from build123d import *

# Parameters (mm, degrees)
BOSS_EXTRUDE1_DEPTH     = 40
CUT_EXTRUDE1_DEPTH      = 40
SKETCH3_W               = 4.376715803
SKETCH3_H               = 7.921330006
BOSS_EXTRUDE2_DEPTH     = 40
CUT_EXTRUDE2_DEPTH      = 78.145313728
CUT_EXTRUDE2_DEPTH_BACK = 78.145313728
CUT_EXTRUDE3_DEPTH      = 40
CUT_EXTRUDE4_DEPTH      = 43.935998882
CUT_EXTRUDE4_DEPTH_BACK = 43.935998882
SKETCH6_R               = 2
CUT_EXTRUDE5_DEPTH      = 5
SKETCH8_R               = 5
CUT_EXTRUDE6_DEPTH      = 5
CUT_EXTRUDE7_START      = -2
SKETCH9_W               = 6.222682415
SKETCH9_H               = 53.403341902
CUT_EXTRUDE7_DEPTH      = 16


with BuildPart() as part:
    # Sketch1 → Boss-Extrude1 (new body)
    with BuildSketch(Plane(origin=(0, 0, 0), x_dir=(1, 0, 0), z_dir=(0, 1, 0))):
        Polygon((-35, 12.5), (-20.56624327, -12.5), (35, -12.5), (35, 12.5), align=None)
    extrude(amount=BOSS_EXTRUDE1_DEPTH)

    # Sketch2 → Cut-Extrude1 (cut)
    with BuildSketch(Plane.XY.offset(12.5)):
        Polygon((-20.56624327, 40), (35, 32.5), (35, 40), align=None)
        Polygon((35, 7.5), (-20.56624327, 0), (35, 0), align=None)
    extrude(amount=-CUT_EXTRUDE1_DEPTH, mode=Mode.SUBTRACT)

    # Sketch3 → Boss-Extrude2 (add)
    with BuildSketch(Plane(origin=(-20.837341226, 0, 12.030444566), x_dir=(0.4999999999999981, 0, 0.8660254037844397), z_dir=(-0.8660254037844398, 0, 0.4999999999999982))):
        with Locations((-10.675795445, 21.421253709)):
            Rectangle(SKETCH3_W, SKETCH3_H)
    extrude(amount=BOSS_EXTRUDE2_DEPTH)

    # Sketch4 → Cut-Extrude2 (cut, two sides: drawn at the far end of the back side and taken through both)
    with BuildSketch(Plane(origin=(-4.243718771, 0, -7.350336525), x_dir=(0.8660254037844397, 0, -0.4999999999999983), z_dir=(0.4999999999999982, 0, 0.8660254037844396)).offset(-CUT_EXTRUDE2_DEPTH_BACK)):
        with BuildLine():
            Line((-25.260889132, 35.934120187), (-19.597573928, 35.934120187))
            ThreePointArc((-19.597573928, 35.934120187), (-17.574079433, 36.729704946), (-16.260889132, 34.996783621))
            Line((-16.260889132, 34.996783621), (-16.260889132, 27.623217913))
            ThreePointArc((-16.260889132, 27.623217913), (-14.610889132, 19.996783621), (-16.260889132, 12.37034933))
            Line((-16.260889132, 12.37034933), (-16.260889132, 4.996783621))
            ThreePointArc((-16.260889132, 4.996783621), (-17.574079433, 3.263862297), (-19.597573928, 4.059447055))
            Line((-19.597573928, 4.059447055), (-25.260889132, 4.059447055))
            Line((-25.260889132, 4.059447055), (-25.260889132, 11.549622397))
            Line((-25.260889132, 11.549622397), (-69.354192402, 11.549622397))
            Line((-69.354192402, 11.549622397), (-69.354192402, 27.546843348))
            Line((-69.354192402, 27.546843348), (-25.260889132, 26.613076168))
            Line((-25.260889132, 26.613076168), (-25.260889132, 35.934120187))
        make_face()
    extrude(amount=CUT_EXTRUDE2_DEPTH + CUT_EXTRUDE2_DEPTH_BACK, mode=Mode.SUBTRACT)

    # Sketch5 → Cut-Extrude3 (cut)
    with BuildSketch(Plane(origin=(0, 0, -12.5), x_dir=(-1, 0, 0), z_dir=(0, 0, -1))):
        with BuildLine():
            Line((-11.141275202, 21.5), (29.874932975, 21.5))
            Line((29.874932975, 21.5), (29.874932975, 18.5))
            Line((29.874932975, 18.5), (-11.142492493, 18.5))
            ThreePointArc((-11.142492493, 18.5), (-26.999999341, 20.006434648), (-11.141275202, 21.5))
        make_face()
    extrude(amount=-CUT_EXTRUDE3_DEPTH, mode=Mode.SUBTRACT)

    # Sketch6 → Cut-Extrude4 (cut, two sides: drawn at the far end of the back side and taken through both)
    with BuildSketch(Plane(origin=(0, 18.5, 0), x_dir=(1, 0, 0), z_dir=(0, 1, 0)).offset(-CUT_EXTRUDE4_DEPTH_BACK)):
        Circle(SKETCH6_R)
    extrude(amount=CUT_EXTRUDE4_DEPTH + CUT_EXTRUDE4_DEPTH_BACK, mode=Mode.SUBTRACT)

    # Sketch7 → Cut-Extrude5 (cut)
    with BuildSketch(Plane.XZ):
        Polygon((1.8525736, 3.461402084), (-2.071375338, 3.335076842), (-3.923948938, -0.126325242), (-1.8525736, -3.461402084), (2.071375338, -3.335076842), (3.923948938, 0.126325242), align=None)
    extrude(amount=-CUT_EXTRUDE5_DEPTH, mode=Mode.SUBTRACT)

    # Sketch8 → Cut-Extrude6 (cut)
    with BuildSketch(Plane(origin=(0, 40, 0), x_dir=(1, 0, 0), z_dir=(0, 1, 0))):
        with Locations(Location((0, 0, 0), (0, 0, 270))):
            Circle(SKETCH8_R)
    extrude(amount=-CUT_EXTRUDE6_DEPTH, mode=Mode.SUBTRACT)

    # Sketch9 → Cut-Extrude7 (cut)
    with BuildSketch(Plane(origin=(-14.082343077, 0, 8.130444566), x_dir=(0.4999999999999982, 0, 0.8660254037844397), z_dir=(-0.8660254037844398, 0, 0.4999999999999983)).offset(CUT_EXTRUDE7_START)):
        with Locations((-26.065813196, 19.047949313)):
            Rectangle(SKETCH9_W, SKETCH9_H)
        Polygon((6.045528012, 45.749620264), (6.045528012, -7.653721638), (13.717164193, -7.653721638), (13.717164193, 42.686575292), (13.717164193, 45.749620264), align=None)
    extrude(amount=CUT_EXTRUDE7_DEPTH, mode=Mode.SUBTRACT)


solid = part.part
For this review, take the finished solid that the model builds, in its own axes (mm). A direction names the side the tool comes from. Round coordinates to 2 decimals unless told otherwise and drop trailing zeros. Write each loop counter-clockwise with the first axis right and the second up, starting at its lowest first coordinate (ties: lowest second). Pieces come first, ordered by that corner, then holes. Notation, with made-up numbers: M 15.25,2.25 L 22.25,2.25 A12 ccw 22.25,13.25 Z; hole C 13.5,-20.5 d9. An arc over 180 degrees is marked long. Write item = value, one per line. Start each with the question number.
(1) We need section B-B (y = 30). Give the boundary of the cut face in (x, z), then the cut area to 3 significant figures.
(2) The part is to be moulded in two halves that separate along X. For faces 4 (the face through (-25, 0, -3)), 5 (the face through (7.6, 3.8, 0.2)), 6 (the face through (-26.523, 37.939, 2.183)), 7 (the face through (-4.88, 36.15, -1.08)), say which applies: +X half, -X half, draft (parallel to the pull), parting line (faces both ways), or undercut.
(3) Clearance check with flat-ended pins moving along their axes: pin 1 Ø6.5 at (x, z) = (0, 0) entering from +Y; pin 2 Ø2 at (x, z) = (1.5, -9.5) entering from -Y; pin 3 Ø12.5 at (x, z) = (-9, 3.5) entering from -Y. State where each tip first meets the part, or that it passes through.
(4) We need section A-A (x = 13). Give the boundary of the cut face in (y, z), then the cut area to 3 significant figures.
(5) For faces 1 (the face through (-17.524, 24.673, 0.074)), 2 (the face through (2, 5, -1)), 3 (the face through (-3, 18.5, 0)), list the 3-axis set-ups (+Z, -Z, +X, -X, +Y, -Y) from which the entire face can be reached by the end or side of a thin tool; tool diameter is ignored.
(6) For line 1 along Z through (x, y) = (0, 27); line 2 along Z through (x, y) = (0, 36.25); line 3 along Y through (x, z) = (9.5, -9.25), list the stretches that pass through material, from the lowest coordinate up.
(7) We need section C-C (x = 0). Give the boundary of the cut face in (y, z).
Results found:
q1.outline = M -25.56,-11.75 L -24.26,-12.5 L 35,-12.5 L 35,12.5 L -9.25,12.5 L -9.33,12.37 L -9.56,12.5 L -11.56,12.5 Z; hole C 0,0 d4
q1.area = 1,330 mm²
q2.face_4 = draft
q2.face_5 = +X half
q2.face_6 = -X half
q2.face_7 = undercut
q3.pin_1 = 35
q3.pin_2 = 2.84
q3.pin_3 = 0.72
q4.outline = M 4.53,-12.5 L 14.71,-12.5 L 14.71,12.5 L 4.53,12.5 Z; M 25.29,-12.5 L 35.47,-12.5 L 35.47,12.5 L 25.29,12.5 Z
q4.area = 509 mm²
q5.face_1 = +Z, -X
q5.face_2 = -Y
q5.face_3 = +Z, -Z, -X
q6.line_1 = -12.5 to -2, 2 to 12.5
q6.line_2 = -12.5 to -5, 5 to 12.5
q6.line_3 = 4.06 to 18.5, 21.5 to 35.94
q7.outline = M 2.78,-12.5 L 18.5,-12.5 L 18.5,-2 L 5,-2 L 5,-3.4 L 2.78,-3.4 Z; M 2.78,3.4 L 5,3.4 L 5,2 L 18.5,2 L 18.5,12.5 L 2.78,12.5 Z; M 21.5,-12.5 L 37.22,-12.5 L 37.22,-5 L 35,-5 L 35,-2 L 21.5,-2 Z; M 21.5,2 L 35,2 L 35,5 L 37.22,5 L 37.22,12.5 L 21.5,12.5 Z
